from build123d import *

# Parameters (mm, degrees)
SKETCH7_R               = 3.45
MAIN_BODY_DEPTH         = 3.5
MATE_HOLE_REACH         = 9.005
MATE_START              = -1
SKETCH9_R               = 2.45
CUT_EXTRUDE2_DEPTH      = 7.004581584
CUT_EXTRUDE2_DEPTH_BACK = 7.004581584
SKETCH10_R              = 0.84
BOSS_EXTRUDE2_DEPTH     = 1.4


with BuildPart() as part:
    # Sketch7 → main body (new body)
    with BuildSketch(Plane.XY):
        Circle(SKETCH7_R)
    extrude(amount=-MAIN_BODY_DEPTH)

    # Sketch9 → mate hole (cut, up to next)
    with BuildSketch(Plane.XY.offset(MATE_START), mode=Mode.PRIVATE) as mate_hole_sk1:
        Circle(SKETCH9_R)
    mate_hole_tool1 = extrude(mate_hole_sk1.sketch, amount=-MATE_HOLE_REACH, mode=Mode.PRIVATE) & part.part
    add(mate_hole_tool1.solids().sort_by_distance((0, 0, -1))[0], mode=Mode.SUBTRACT)

    # Sketch10 → Cut-Extrude2 (cut, two sides: drawn at the far end of the back side and taken through both)
    with BuildSketch(Plane.XY.offset(-CUT_EXTRUDE2_DEPTH_BACK)):
        Circle(SKETCH10_R)
    extrude(amount=CUT_EXTRUDE2_DEPTH + CUT_EXTRUDE2_DEPTH_BACK, mode=Mode.SUBTRACT)

    # Sketch11 → Boss-Extrude2 (add)
    with BuildSketch(Plane.XY):
        with BuildLine():
            Line((-3.235641734, 1.197130973), (-9.007776393, 0.556197651))
            ThreePointArc((-9.007776393, 0.556197651), (-9.505632664, 0), (-9.007776393, -0.556197651))
            Line((-9.007776393, -0.556197651), (-3.235641734, -1.197130973))
            ThreePointArc((-3.235641734, -1.197130973), (-3.45, 0), (-3.235641734, 1.197130973))
        make_face()
    extrude(amount=-BOSS_EXTRUDE2_DEPTH)


solid = part.part
The listing builds one solid part. Answer for the finished solid, in the listing's coordinates (mm). A direction names the side the tool comes from. Coordinates: 2 decimals unless noted, no trailing zeros. Write each loop counter-clockwise with the first axis right and the second up, starting at its lowest first coordinate (ties: lowest second). Pieces come first, ordered by that corner, then holes. Notation, with made-up numbers: (64.25, -30) - (102.25, -30) arc R22 ccw to (102.25, -16) - close; hole circle Ø6 at (61, -35.5). An arc over 180 degrees is marked (long way). Return JSON: item names as keys, results as strings.
1. For a pull along Y with two mould halves and no side action, classify faces 1 (the face through (0.388, -0.745, -0.507)), 2 (the face through (-6.08, 0.88, -0.69)), 3 (the face through (-6.162, -0.872, -0.69)) as +Y half, -Y half, draft (parallel to the pull), parting line (faces both ways), or undercut.
Final values:
{"face 1": "undercut", "face 2": "+Y half", "face 3": "-Y half"}
2. The part is cut by section B-B on x = 0. Determine the outline of the cut face in (y, z), then the cut area to 3 significant figures.
Final values:
{"outline": "(-3.45, -3.5) - (-2.45, -3.5) - (-2.45, -1) - (-0.84, -1) - (-0.84, 0) - (-3.45, 0) - close; (0.84, -1) - (2.45, -1) - (2.45, -3.5) - (3.45, -3.5) - (3.45, 0) - (0.84, 0) - close", "area": "10.2 mm^2"}
3. Which of the six approach directions +Z, -Z, +X, -X, +Y, -Y give full straight-line access (tool end or side, diameter ignored) to faces 4 (the face through (1, 0, -1)), 5 (the face through (1.5, -2.3, -3.5))?
Final values:
{"face 4": "-Z", "face 5": "-Z, +X, -X, +Y, -Y"}
4. Each of these flat-tipped pins is pushed along its axis until it touches: pin 1 Ø0.7 at (x, y) = (-7, 0.5) entering from -Z; pin 2 Ø2 at (x, y) = (-4, -1.5) entering from -Z; pin 3 Ø2.5 at (x, y) = (0.5, -0.5) entering from -Z; pin 4 Ø1.5 at (x, z) = (-7, -2) entering from -Y. Where does it stop, or does it pass through?
Final values:
{"pin 1": "z = -1.4", "pin 2": "z = -3.5", "pin 3": "z = -1", "pin 4": "y = -0.83"}
5. Consider line 1 along Y through (x, z) = (0, -1.6); line 2 along Y through (x, z) = (0, -0.65); line 3 along Z through (x, y) = (-4, -0.75). Determine where each line is inside the solid, lowest interval first.
Final values:
{"line 1": "-3.45 to -2.45, 2.45 to 3.45", "line 2": "-3.45 to -0.84, 0.84 to 3.45", "line 3": "-1.4 to 0"}
6. The part is cut by section D-D on y = -2. Determine the outline of the cut face in (x, z), then the cut area to 3 significant figures.
Final values:
{"outline": "(-2.81, -3.5) - (-1.42, -3.5) - (-1.42, -1) - (1.42, -1) - (1.42, -3.5) - (2.81, -3.5) - (2.81, 0) - (-2.81, 0) - close", "area": "12.6 mm^2"}
7. The part is cut by section A-A on y = 0. Determine the outline of the cut face in (x, z), then the cut area to 3 significant figures.
Final values:
{"outline": "(-9.51, -1.4) - (-3.45, -1.4) - (-3.45, -3.5) - (-2.45, -3.5) - (-2.45, -1) - (-0.84, -1) - (-0.84, 0) - (-9.51, 0) - close; (0.84, -1) - (2.45, -1) - (2.45, -3.5) - (3.45, -3.5) - (3.45, 0) - (0.84, 0) - close", "area": "18.7 mm^2"}
8. The part is cut by section C-C on z = -1.7. Determine the outline of the cut face in (x, y), then the cut area to 3 significant figures.
Final values:
{"outline": "circle Ø6.9 at (0, 0); hole circle Ø4.9 at (0, 0)", "area": "18.5 mm^2"}
